```python
from build123d import *

# Parameters (mm, degrees)
SKETCH1_R               = 7.15
SKETCH1_R_2             = 5
BOSS_EXTRUDE1_DEPTH     = 10
CUT_EXTRUDE1_DEPTH      = 15.221286862
CUT_EXTRUDE1_DEPTH_BACK = 15.221286862
SKETCH2_R               = 8.28
BOSS_EXTRUDE2_START     = 1
SKETCH3_R               = 7.15
SKETCH3_R_2             = 5
BOSS_EXTRUDE2_DEPTH     = 1


with BuildPart() as part:
    # Sketch1 → Boss-Extrude1 (new body)
    with BuildSketch(Plane(origin=(0, 0, 0), x_dir=(1, 0, 0), z_dir=(0, 1, 0))):
        with Locations(Location((0, 0, 0), (0, 0, 270))):
            Circle(SKETCH1_R)
        with Locations(Location((0, 0, 0), (0, 0, 270))):
            Circle(SKETCH1_R_2, mode=Mode.SUBTRACT)
    extrude(amount=BOSS_EXTRUDE1_DEPTH)

    # Sketch2 → Cut-Extrude1 (cut, two sides: drawn at the far end of the back side and taken through both)
    with BuildSketch(Plane.XY.offset(-CUT_EXTRUDE1_DEPTH_BACK)):
        with Locations((0, 9.28)):
            Circle(SKETCH2_R)
    extrude(amount=CUT_EXTRUDE1_DEPTH + CUT_EXTRUDE1_DEPTH_BACK, mode=Mode.SUBTRACT)

    # Sketch3 → Boss-Extrude2 (add)
    with BuildSketch(Plane.XZ.offset(BOSS_EXTRUDE2_START)):
        with Locations(Location((0, 0, 0), (0, 0, 270))):
            Circle(SKETCH3_R)
        with Locations(Location((0, 0, 0), (0, 0, 270))):
            Circle(SKETCH3_R_2, mode=Mode.SUBTRACT)
    extrude(amount=-BOSS_EXTRUDE2_DEPTH)


solid = part.part
```
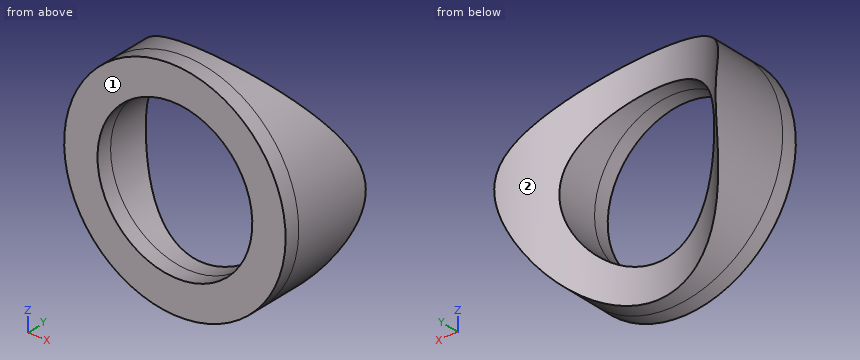
Work out the finished part from the listing and answer in its coordinate system (mm). Face numbers are marked on the shaded views. Give positions to 0.01 mm unless a question says otherwise; leave off trailing zeros. Loops run counter-clockwise (first coordinate to the right, second up) from the corner with the lowest first, then second, coordinate; pieces in that order, holes last. Notation, with made-up numbers: (24, 1) -> (66, 1) arc R20 ccw to (66, 8) -> close; hole circle Ø6 at (-23.5, 89). An arc over 180 degrees is marked (long way). One line per question, with ' | ' between items. Start each with the question number.
1) Section D-D, the plane y = 0.75 is taken. Determine the outline of the cut face in (x, z), then the cut area to 3 significant figures.
2) Determine the mould class of the marked faces 1 and 2 for opening direction X: +X half, -X half, draft (parallel to the pull), parting line (faces both ways), or undercut.
3) Section C-C, the plane y = 3.25 is taken. Determine the outline of the cut face in (x, z), then the cut area to 3 significant figures.
4) Section A-A, the plane x = 0 is taken. Determine the outline of the cut face in (y, z), then the cut area to 3 significant figures.
5) Section B-B, the plane z = -3 is taken. Determine the outline of the cut face in (x, y), then the cut area to 3 significant figures.
6) Each of these flat-tipped pins is pushed along its axis until it touches: pin 1 (1.5 mm diameter, centred on x = -1.5, y = 3, fed in from +Z); pin 2 (1 mm diameter, centred on y = 0, z = 1.5, fed in from -X). Where does it stop, or does it pass through?
7) Straight lines are drawn through the part: L1, parallel to X at y = 0.95, z = 0; L2, parallel to Z at x = 2.75, y = 1.25. For each, find the intervals that lie inside material, in ascending order.
Resolved:
1) outline: circle Ø14.3 at (0, 0); hole circle Ø10 at (0, 0) | area: 82.1 mm2
2) face 1: draft | face 2: undercut
3) outline: (-5.67, -4.35) -> (-5.67, 4.35) arc R7.15 ccw to start; (5.67, -4.35) arc R7.15 ccw to (5.67, 4.35) -> close | area: 17.5 mm2
4) outline: (-1, -7.15) -> (1, -7.15) -> (1, -5) -> (-1, -5) -> close; (-1, 5) -> (1, 5) -> (1, 7.15) -> (-1, 7.15) -> close | area: 8.60 mm2
5) outline: (-6.49, -1) -> (-4, -1) -> (-4, 2.03) arc R8.28 cw to (-6.49, 4.14) -> close; (4, -1) -> (6.49, -1) -> (6.49, 4.14) arc R8.28 cw to (4, 2.03) -> close | area: 19.6 mm2
6) pin 1: through | pin 2: x = -7.08
7) L1: -7.15 to -5, 5 to 7.15 | L2: -6.6 to -4.18, 4.18 to 6.6
